The model under review builds one solid part; all positions refer to its coordinate system, in mm. A direction names the side the tool comes from. Round coordinates to 2 decimals unless told otherwise and drop trailing zeros. Order: outer loops, then holes, each group sorted by start corner. A loop starts at its lowest first (then second) coordinate and runs counter-clockwise, first axis right, second up. Notation, with made-up numbers: M 13.25,33 L 52.25,33 A13 cw 52.25,58 Z; hole C 71,40 d2. An arc over 180 degrees is marked long. Answer as a JSON object with one key per item and string values. Group by question number.
1. Machinability: for faces 1 (the face through (-6.5, 11, 1)), 2 (the face through (-12.5, -13, 1)), 3 (the face through (1, 5, 1)), which of the approach directions +Z, -Z, +X, -X, +Y, -Y give a long, thin tool a straight path to every point of the face, cutting with its end or side? Answer none if there is none.
2. Add section B-B on x = 9.5. State the section outline as (y, z) points, and give its area (3 significant figures).
3. Add section A-A on x = 3. State the section outline as (y, z) points, and give its area (3 significant figures).
4. Add section D-D on y = -44. State the section outline as (x, z) points, and give its area (3 significant figures).
5. Mouldability with a two-part tool opening along X and no side actions: class faces 4 (the face through (0, 1, 1)), 5 (the face through (4.5, -60, 1)), 6 (the face through (9, 12.5, 1)) as released by +X, released by -X, zero draft, split by the parting line, or undercut.
6. To check wall thickness, follow probe 1 along Y at (x, z) = (6.5, 0.35); probe 2 along Y at (x, z) = (3.25, 0.35); probe 3 along Y at (x, z) = (0.25, 2.4). State the ranges of each line that lie inside material, in increasing order. Write a range as [from, to].
7. Clearance check with flat-ended pins moving along their axes: P1, Ø1.5, axis at y = -28, z = 2, coming from the +X side; P2, Ø1.5, axis at y = 10.5, z = 1, coming from the -X side; P3, Ø0.8, axis at x = -3.5, z = 2, coming from the +Y side. State where each tip first meets the part, or that it passes through.
8. Add section C-C on z = 2. State the section outline as (x, y) points, and give its area (3 significant figures).
```python
from build123d import *

# Parameters (mm, degrees)
F0_W     = 4
F0_H     = 4
F0_W_2   = 6
F0_H_2   = 34
F0_W_3   = 10
F0_H_3   = 25
F1_DEPTH = 3


with BuildPart() as f1:
    # F0 (on Top) → F1 (new body)
    with BuildSketch(Plane.XY):
        with Locations((-14.5, -40.5)):
            Rectangle(F0_W, F0_H)
        with Locations((7.5, -59.5)):
            Rectangle(F0_W_2, F0_H_2)
        with Locations((-7.5, -25)):
            Rectangle(F0_W_3, F0_H_3)
        Polygon((10.5, -37.5), (-2.5, -37.5), (-12.5, -37.5), (-12.5, -38.5), (-12.5, -42.5), (4.5, -42.5), (10.5, -42.5), align=None)
        Polygon((12.5, -12.5), (12.5, 12.5), (4.5, 12.5), (4.5, 9.5), (0, 9.5), (0, 5.5), (1, 5.5), (1, 3.5), (0, 3.5), (0, -1.5), (-3, -1.5), (-3, 3.5), (-4, 3.5), (-4, 5.5), (-3, 5.5), (-3, 9.5), (-6.5, 9.5), (-6.5, 12.5), (-12.5, 12.5), (-12.5, -12.5), (-2.5, -12.5), align=None)
    extrude(amount=F1_DEPTH)


solid = f1.part
```
Recorded:
{
 "1": {"face 1": "+Z, -Z, +Y", "face 2": "+Z, -Z, -X, +Y", "face 3": "+Z, -Z"},
 "2": {"outline": "M -76.5,0 L -37.5,0 L -37.5,3 L -76.5,3 Z; M -12.5,0 L 12.5,0 L 12.5,3 L -12.5,3 Z", "area": "192 mm²"},
 "3": {"outline": "M -42.5,0 L -37.5,0 L -37.5,3 L -42.5,3 Z; M -12.5,0 L 9.5,0 L 9.5,3 L -12.5,3 Z", "area": "81.0 mm²"},
 "4": {"outline": "M 4.5,0 L 10.5,0 L 10.5,3 L 4.5,3 Z", "area": "18.0 mm²"},
 "5": {"face 4": "undercut", "face 5": "released by -X", "face 6": "zero draft"},
 "6": {"probe 1": "y = [-76.5, -37.5], [-12.5, 12.5]", "probe 2": "y = [-42.5, -37.5], [-12.5, 9.5]", "probe 3": "y = [-42.5, -37.5], [-12.5, 3.5], [5.5, 9.5]"},
 "7": {"P1": "stops at x = -2.5", "P2": "stops at x = -12.5", "P3": "stops at y = 9.5"},
 "8": {"outline": "M -16.5,-42.5 L 4.5,-42.5 L 4.5,-76.5 L 10.5,-76.5 L 10.5,-37.5 L -2.5,-37.5 L -2.5,-12.5 L 12.5,-12.5 L 12.5,12.5 L 4.5,12.5 L 4.5,9.5 L 0,9.5 L 0,5.5 L 1,5.5 L 1,3.5 L 0,3.5 L 0,-1.5 L -3,-1.5 L -3,3.5 L -4,3.5 L -4,5.5 L -3,5.5 L -3,9.5 L -6.5,9.5 L -6.5,12.5 L -12.5,12.5 L -12.5,-38.5 L -16.5,-38.5 Z", "area": "1,140 mm²"}
}
